Part model, mm, in its own coordinate system. Round coordinates to 2 decimals unless told otherwise and drop trailing zeros. Loops run counter-clockwise (first coordinate to the right, second up) from the corner with the lowest first, then second, coordinate; pieces in that order, holes last.
1) Drop flat-ended pins along their axis: P1, Ø3, axis at y = 2, z = -17, coming from the +X side; P2, Ø1.2, axis at x = 8.5, z = 11.5, coming from the +Y side; P3, Ø1.2, axis at x = -9, z = -10.5, coming from the -Y side; P4, Ø1.9, axis at x = 7.5, y = 0, coming from the +Z side. Give the stop position or say it passes through.
2) Band-saw the part on A-A, the plane z = -14. Write the cut outline in (x, y).
3) Band-saw the part on B-B, the plane y = -2.25. Write the cut outline in (x, z).
4) Probe line 1 (X direction, y = 0, z = 1); line 2 (Z direction, x = 8.75, y = -2.5); line 3 (Y direction, x = -7.5, z = 2.5). List the from-to ranges inside material, lowest first.
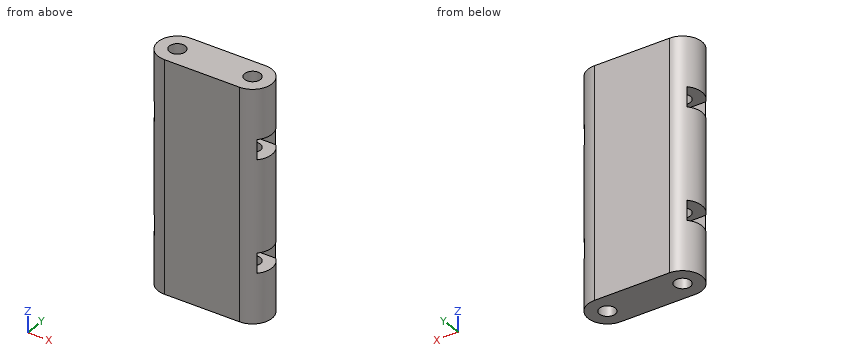
Autodesk Inventor part; units mm, degrees
ref_plane "Work Plane1" through (0, 0, 13.25) normal (0, 0, 1) x (1, 0, 0)
ref_plane "YZ Plane" through (0, 0, 0) normal (1, 0, 0) x (0, 1, 0)
ref_plane "XZ Plane" through (0, 0, 0) normal (0, 1, 0) x (-1, 0, 0)
sketch "Sketch1" plane through (0, 0, 0) normal (0, 0, 1) x (1, 0, 0)
  line L0 (-7.5, 0) -> (7.5, 0) construction
  line L1 (-7.5, -3.9) -> (7.5, -3.9)
  line L2 (7.5, 3.9) -> (-7.5, 3.9)
  arc A0 (-7.5, 3.9) -> (-7.5, -3.9) centre (-7.5, 0) ccw
  arc A1 (7.5, -3.9) -> (7.5, 3.9) centre (7.5, 0) ccw
  point P0 (0, 0)
  point P1 (0, 0)
  dimension "d0" = 3.9
  dimension "d1" = 15
extrude "Extrusion1" add sketch "Sketch1" along normal mid plane 46.5
sketch "Sketch2" plane through (0, 0, 23.25) normal (0, 0, 1) x (1, 0, 0)
  arc A0 (-7.5, 3.9) -> (-7.5, -3.9) centre (-7.5, 0) ccw
  arc A1 (7.5, -3.9) -> (7.5, 3.9) centre (7.5, 0) ccw
  point P0 (0, 0)
hole "Hole1" at (-7.5, 0, 23.25) at (7.5, 0, 23.25) direction (0, 0, -1) diameter 3.2 end through all
ref_plane "Work Plane1" through (0, 0, 13.25) normal (0, 0, 1) x (1, 0, 0)
sketch "Sketch3" plane through (0, 0, 13.25) normal (0, 0, 1) x (1, 0, 0)
  circle A0 centre (-7.5, 0) radius 1.6
  line L0 (-9.0877, 2.75) -> (-5.9123, 2.75)
  line L1 (-5.9123, 2.75) -> (-4.3246, 0)
  line L2 (-4.3246, 0) -> (-5.9123, -2.75)
  line L3 (-5.9123, -2.75) -> (-9.0877, -2.75)
  line L4 (-9.0877, -2.75) -> (-10.6754, 0)
  line L5 (-10.6754, 0) -> (-9.0877, 2.75)
  line L6 (-9.0877, 2.75) -> (-10.2654, 2.75)
  arc A1 (-7.5, 3.9) -> (-7.5, -3.9) centre (-7.5, 0) ccw
  line L7 (-9.0877, -2.75) -> (-10.2654, -2.75)
  point P0 (0, 0)
  dimension "d12" = 5.5
extrude "Extrusion2" cut sketch "Sketch3" against normal blind 4
mirror "Mirror1" about plane through (0, 0, 0) normal (1, 0, 0) of "Extrusion2"
mirror "Mirror2" about plane through (0, 0, 0) normal (0, 0, 1) of "Extrusion2", "Mirror1"
properties part number "Standoff" material "PET Plastic"
Reported:
1. P1: stops at x = 11.37
1. P2: stops at y = 3.88
1. P3: stops at y = -3.79
1. P4: passes through
2. outline: (-7.5, -3.9) - (7.5, -3.9) arc R3.9 ccw to (7.5, 3.9) - (-7.5, 3.9) arc R3.9 ccw to start; hole circle Ø3.2 at (-7.5, 0); hole circle Ø3.2 at (7.5, 0)
3. outline: (-10.69, -23.25) - (10.69, -23.25) - (10.69, -13.25) - (5.62, -13.25) - (5.62, -9.25) - (10.69, -9.25) - (10.69, 9.25) - (5.62, 9.25) - (5.62, 13.25) - (10.69, 13.25) - (10.69, 23.25) - (-10.69, 23.25) - (-10.69, 13.25) - (-5.62, 13.25) - (-5.62, 9.25) - (-10.69, 9.25) - (-10.69, -9.25) - (-5.62, -9.25) - (-5.62, -13.25) - (-10.69, -13.25) - close
4. line 1: x = -11.4 to -9.1, -5.9 to 5.9, 9.1 to 11.4
4. line 2: z = -23.25 to -13.25, -9.25 to 9.25, 13.25 to 23.25
4. line 3: y = -3.9 to -1.6, 1.6 to 3.9
